```python
from build123d import *

# Parameters (mm, degrees)
SKETCH_1_W      = 43.5
SKETCH_1_H      = 21
SKETCH_1_R      = 4
SKETCH_1_R_2    = 0.75
SKETCH_1_R_3    = 1.75
SKETCH_1_W_2    = 12
SKETCH_1_H_2    = 12
SKETCH_1_W_3    = 9.5
SKETCH_1_H_3    = 8.5
SKETCH_1_H_4    = 4.5
EXTRUDE_1_DEPTH = 1
SKETCH_1_3_R    = 4
EXTRUDE_2_DEPTH = 11
SKETCH_1_4_W    = 9.5
SKETCH_1_4_H    = 8.5
EXTRUDE_3_DEPTH = 5
SKETCH_1_5_W    = 9.5
SKETCH_1_5_H    = 4.5
EXTRUDE_4_DEPTH = 10
SKETCH_1_6_W    = 12
SKETCH_1_6_H    = 12
EXTRUDE_5_DEPTH = 8
SKETCH_2_R      = 1
EXTRUDE_6_DEPTH = 2


with BuildPart() as part:
    # Sketch 1 → Extrude 1 (new body)
    # profile 1 of 8: a face of its own
    with BuildSketch(Plane(origin=(0, 0, 0), x_dir=(1, 0, 0), z_dir=(0, 1, 0))):
        Rectangle(SKETCH_1_W, SKETCH_1_H)
        with Locations((16.75, 0)):
            Circle(SKETCH_1_R, mode=Mode.SUBTRACT)
        with Locations((-16.75, 0)):
            Circle(SKETCH_1_R, mode=Mode.SUBTRACT)
        with Locations(Location((-20, -8.75, 0), (0, 0, 270))):
            Circle(SKETCH_1_R_2, mode=Mode.SUBTRACT)
        with Locations(Location((20, -8.75, 0), (0, 0, 270))):
            Circle(SKETCH_1_R_2, mode=Mode.SUBTRACT)
        with Locations(Location((20, 8.75, 0), (0, 0, 270))):
            Circle(SKETCH_1_R_2, mode=Mode.SUBTRACT)
        with Locations(Location((-20, 8.75, 0), (0, 0, 270))):
            Circle(SKETCH_1_R_2, mode=Mode.SUBTRACT)
        with Locations((15, -7.75)):
            Circle(SKETCH_1_R_3, mode=Mode.SUBTRACT)
        with Locations((-15, 7.75)):
            Circle(SKETCH_1_R_3, mode=Mode.SUBTRACT)
        with Locations((-5.75, 3.5)):
            Rectangle(SKETCH_1_W_2, SKETCH_1_H_2, mode=Mode.SUBTRACT)
        with Locations((7, -4.25)):
            Rectangle(SKETCH_1_W_3, SKETCH_1_H_3, mode=Mode.SUBTRACT)
        with Locations((-7, -7.25)):
            Rectangle(SKETCH_1_W_3, SKETCH_1_H_4, mode=Mode.SUBTRACT)
    # profile 2 of 8: a face of its own
    with BuildSketch(Plane(origin=(0, 0, 0), x_dir=(1, 0, 0), z_dir=(0, 1, 0))):
        with Locations((-16.75, 0)):
            Circle(SKETCH_1_R)
    # profile 3 of 8: a face of its own
    with BuildSketch(Plane(origin=(0, 0, 0), x_dir=(1, 0, 0), z_dir=(0, 1, 0))):
        with Locations((-5.75, 3.5)):
            Rectangle(SKETCH_1_W_2, SKETCH_1_H_2)
    # profile 4 of 8: a face of its own
    with BuildSketch(Plane(origin=(0, 0, 0), x_dir=(1, 0, 0), z_dir=(0, 1, 0))):
        with Locations((-7, -7.25)):
            Rectangle(SKETCH_1_W_3, SKETCH_1_H_4)
    # profile 5 of 8: a face of its own
    with BuildSketch(Plane(origin=(0, 0, 0), x_dir=(1, 0, 0), z_dir=(0, 1, 0))):
        with Locations((7, -4.25)):
            Rectangle(SKETCH_1_W_3, SKETCH_1_H_3)
    # profile 6 of 8: a face of its own
    with BuildSketch(Plane(origin=(0, 0, 0), x_dir=(1, 0, 0), z_dir=(0, 1, 0))):
        with Locations((15, -7.75)):
            Circle(SKETCH_1_R_3)
    # profile 7 of 8: a face of its own
    with BuildSketch(Plane(origin=(0, 0, 0), x_dir=(1, 0, 0), z_dir=(0, 1, 0))):
        with Locations((16.75, 0)):
            Circle(SKETCH_1_R)
    # profile 8 of 8: a face of its own
    with BuildSketch(Plane(origin=(0, 0, 0), x_dir=(1, 0, 0), z_dir=(0, 1, 0))):
        with Locations((-15, 7.75)):
            Circle(SKETCH_1_R_3)
    extrude(amount=-EXTRUDE_1_DEPTH)

    # Sketch 1_3 → Extrude 2 (add)
    with BuildSketch(Plane(origin=(0, 0, 0), x_dir=(1, 0, 0), z_dir=(0, 1, 0))):
        with Locations(Location((-16.75, 0, 0), (0, 0, 270))):
            Circle(SKETCH_1_3_R)
        with Locations(Location((16.75, 0, 0), (0, 0, 270))):
            Circle(SKETCH_1_3_R)
    extrude(amount=EXTRUDE_2_DEPTH)

    # Sketch 1_4 → Extrude 3 (add)
    with BuildSketch(Plane(origin=(0, 0, 0), x_dir=(1, 0, 0), z_dir=(0, 1, 0))):
        with Locations((7, -4.25)):
            Rectangle(SKETCH_1_4_W, SKETCH_1_4_H)
    extrude(amount=EXTRUDE_3_DEPTH)

    # Sketch 1_5 → Extrude 4 (add)
    with BuildSketch(Plane(origin=(0, 0, 0), x_dir=(1, 0, 0), z_dir=(0, 1, 0))):
        with Locations((-7, -7.25)):
            Rectangle(SKETCH_1_5_W, SKETCH_1_5_H)
    extrude(amount=EXTRUDE_4_DEPTH)

    # Sketch 1_6 → Extrude 5 (add)
    with BuildSketch(Plane(origin=(0, 0, 0), x_dir=(1, 0, 0), z_dir=(0, 1, 0))):
        with Locations((-5.75, 3.5)):
            Rectangle(SKETCH_1_6_W, SKETCH_1_6_H)
    extrude(amount=EXTRUDE_5_DEPTH)

    # Sketch 2 → Extrude 6 (add)
    with BuildSketch(Plane(origin=(0, 10, 0), x_dir=(1, 0, 0), z_dir=(0, 1, 0))):
        with Locations(Location((-3.25, -8.5, 0), (0, 0, 270))):
            Circle(SKETCH_2_R)
    extrude(amount=EXTRUDE_6_DEPTH)


solid = part.part
```
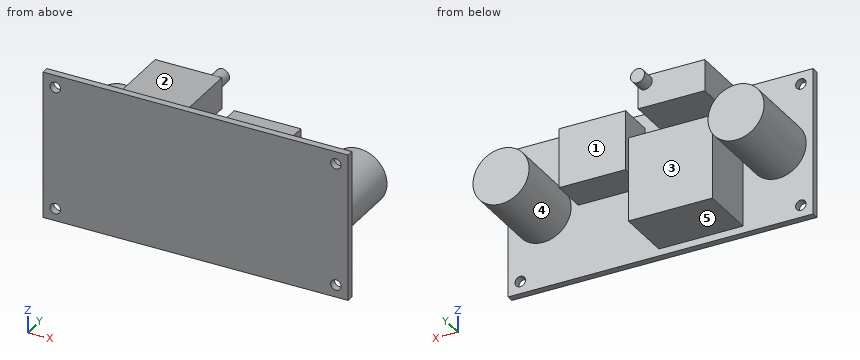
Work out the finished part from the listing and answer in its coordinate system (mm). Face numbers are marked on the shaded views. A direction names the side the tool comes from. Coordinates: 2 decimals unless noted, no trailing zeros. Loops run counter-clockwise (first coordinate to the right, second up) from the corner with the lowest first, then second, coordinate; pieces in that order, holes last.
1) Section D-D (x = 20) is taken. Give the vertices of the cut face in (y, z), plus the area to 3 significant figures.
Results:
outline: (-1, -10.5) - (0, -10.5) - (0, -9.5) - (-1, -9.5) - close; (-1, -8) - (0, -8) - (0, -2.33) - (11, -2.33) - (11, 2.33) - (0, 2.33) - (0, 8) - (-1, 8) - close; (-1, 9.5) - (0, 9.5) - (0, 10.5) - (-1, 10.5) - close
area: 69.3 mm2
2) Flat-ended cylindrical pins translate along their axes: pin 1 (2 mm diameter, centred on x = -20, z = -8.75, fed in from -Y); pin 2 (10 mm diameter, centred on x = -5.5, z = 1, fed in from +Y); pin 3 (2.5 mm diameter, centred on x = -20, z = 8.75, fed in from +Y); pin 4 (6.5 mm diameter, centred on x = -6, y = 3.5, fed in from -Z). Find the tip coordinate at first contact, or state that the pin passes through.
Results:
pin 1: stops at y = -1
pin 2: stops at y = 10
pin 3: stops at y = 0
pin 4: stops at z = -9.5
3) Section C-C (y = 6.5) is taken. Give the vertices of the cut face in (x, z), plus the area to 3 significant figures.
Results:
outline: circle Ø8 at (-16.75, 0); (-11.75, -9.5) - (0.25, -9.5) - (0.25, 2.5) - (-11.75, 2.5) - close; (-11.75, 5) - (-2.25, 5) - (-2.25, 9.5) - (-11.75, 9.5) - close; circle Ø8 at (16.75, 0)
area: 287 mm2
4) Section B-B (x = -7) is taken. Give the vertices of the cut face in (y, z).
Results:
outline: (-1, -10.5) - (0, -10.5) - (0, -9.5) - (8, -9.5) - (8, 2.5) - (0, 2.5) - (0, 5) - (10, 5) - (10, 9.5) - (0, 9.5) - (0, 10.5) - (-1, 10.5) - close
5) For the marked faces 1, 2, 3, 4 and 5, determine the directions among +Z, -Z, +X, -X, +Y, -Y from which every point of the face is accessible in a straight line to the end or side of a thin tool.
Results:
face 1: +Z, -Z, +Y
face 2: +Z, +X, -X, +Y
face 3: -Z, +Y
face 4: +Y
face 5: -Z, +X, -X, +Y
6) Section A-A (z = -8.75) is taken. Give the vertices of the cut face in (x, y).
Results:
outline: (-21.75, -1) - (-20.75, -1) - (-20.75, 0) - (-21.75, 0) - close; (-19.25, -1) - (19.25, -1) - (19.25, 0) - (0.25, 0) - (0.25, 8) - (-11.75, 8) - (-11.75, 0) - (-19.25, 0) - close; (20.75, -1) - (21.75, -1) - (21.75, 0) - (20.75, 0) - close
7) Consider probe 1 along X at (y, z) = (-0.6, -8.75); probe 2 along X at (y, z) = (6.5, -1); probe 3 along Y at (x, z) = (-7, -7). Determine where each line is inside the solid, lowest interval first.
Results:
probe 1: x = -21.75 to -20.75, -19.25 to 19.25, 20.75 to 21.75
probe 2: x = -20.62 to -12.88, -11.75 to 0.25, 12.88 to 20.62
probe 3: y = -1 to 8
